Design review of the part shown in the three views and the two pictorial views. Dimensions are in mm from the part's minimum x, y and z. Round coordinates to 2 decimals unless told otherwise and drop trailing zeros. Write each loop counter-clockwise with the first axis right and the second up, starting at its lowest first coordinate (ties: lowest second). Pieces come first, ordered by that corner, then holes. Notation, with made-up numbers: (43, -6) -> (86, -6) arc R11 ccw to (86, 9) -> close; hole circle Ø2 at (55.25, 56.25). An arc over 180 degrees is marked (long way). Return JSON: item names as keys, results as strings. Group by question number.
1. Take a section at D-D, the plane z = 34.5. Write out the cut boundary in (x, y), then the cut area to 3 significant figures.
2. Take a section at C-C, the plane y = 11. Write out the cut boundary in (x, z), then the cut area to 3 significant figures.
3. Mouldability with a two-part tool opening along Y and no side actions: class the marked faces 1, 2 and 3 as pulls with the +Y half, pulls with the -Y half, needs draft (parallel to the pull), parting line crosses it, or undercut.
4. For line 1 along X through (y, z) = (11, 23); line 2 along Z through (x, y) = (49, 14.75); line 3 along Z through (x, y) = (30.5, 18.75), list the stretches that pass through material, from the lowest coordinate up. Write a range as from..to.
5. Clearance check with flat-ended pins moving along their axes: P1, Ø1.8, axis at y = 10.5, z = 26.5, coming from the +X side; P2, Ø2, axis at x = 56.5, y = 12.5, coming from the -Z side; P3, Ø8, axis at y = 16, z = 28, coming from the -X side; P4, Ø10, axis at x = 71.5, y = 14, coming from the +Z side. State where each tip first meets the part, or that it passes through.
6. Take a section at B-B, the plane x = 109. Write out the cut boundary in (y, z).
7. Take a section at A-A, the plane x = 23. Write out the cut boundary in (y, z).
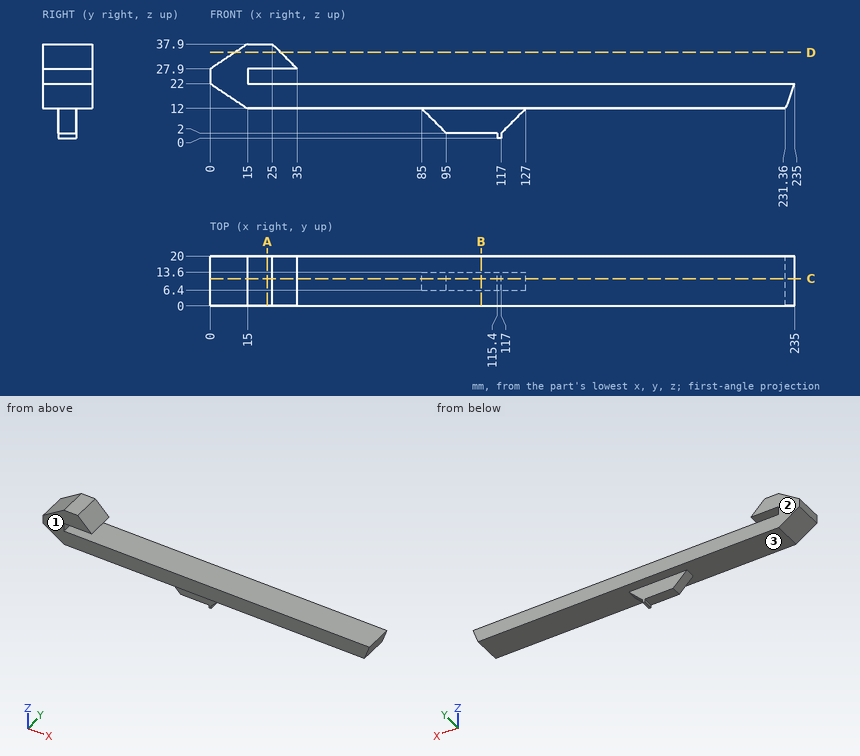
Output:
{
 "1": {"outline": "(9.9, 0) -> (28.4, 0) -> (28.4, 20) -> (9.9, 20) -> close", "area": "370 mm^2"},
 "2": {"outline": "(0, 22) -> (15, 12) -> (85, 12) -> (95, 2) -> (115.4, 2) -> (115.4, 0) -> (117, 0) -> (117, 2) -> (127, 12) -> (231.36, 12) -> (235, 22) -> (15, 22) -> (15, 27.9) -> (35, 27.9) -> (25, 37.9) -> (15, 37.9) -> (0, 27.9) -> close", "area": "2,890 mm^2"},
 "3": {"face 1": "pulls with the -Y half", "face 2": "pulls with the +Y half", "face 3": "needs draft"},
 "4": {"line 1": "x = 0..15", "line 2": "z = 12..22", "line 3": "z = 12..22, 27.9..32.4"},
 "5": {"P1": "stops at x = 15", "P2": "stops at z = 12", "P3": "stops at x = 0", "P4": "stops at z = 22"},
 "6": {"outline": "(0, 12) -> (6.4, 12) -> (6.4, 2) -> (13.6, 2) -> (13.6, 12) -> (20, 12) -> (20, 22) -> (0, 22) -> close"},
 "7": {"outline": "(0, 12) -> (20, 12) -> (20, 22) -> (0, 22) -> close; (0, 27.9) -> (20, 27.9) -> (20, 37.9) -> (0, 37.9) -> close"}
}
